Here's how the part is built. I have some questions about the finished solid (model axes, mm). Give positions to 0.01 mm unless a question says otherwise; leave off trailing zeros. Loops run counter-clockwise (first coordinate to the right, second up) from the corner with the lowest first, then second, coordinate; pieces in that order, holes last.
Q1. We'd pull the mould along Y, two halves only. Please class faces 1 (the face through (-1.5, 0.07, 1.97)), 2 (the face through (-5, 0, 4)), 3 (the face through (-1.08, -4.88, 1.53)): +Y half, -Y half, draft (parallel to the pull), parting line (faces both ways), or undercut.
Q2. I need wall thicknesses on line 1 (Y direction, x = 0, z = 3.8); line 2 (Y direction, x = 0, z = 2.75); line 3 (Y direction, x = -0.5, z = 1.2). Which ranges of each line are inside material? Lowest first, please.
Q3. If we section it at B-B (z = 3.25): Please give me the cut outline in (x, y), plus the area to 3 significant figures.
Q4. If we section it at A-A (z = 1.8): Please give me the cut outline in (x, y), plus the area to 3 significant figures.
from build123d import *

# Parameters (mm, degrees)
F0_R     = 2
F0_R_2   = 1.5
F1_DEPTH = 0.25
F0_R_3   = 5
F0_R_4   = 4.5
F2_R     = 5
F2_R_2   = 4.5
F2_R_3   = 2
F2_R_4   = 1.5
F3_DEPTH = 2.75
F4_R     = 5.75
F4_R_2   = 5
F4_R_3   = 1.5
F5_DEPTH = 0.75
F6_R     = 5.75
F6_R_2   = 4.5
F6_R_3   = 2
F6_R_4   = 1.5
F7_DEPTH = 0.25
F8_SIZE  = 0.1


with BuildPart() as f1:
    # F0 (on Top) → F1 (new body)
    with BuildSketch(Plane.XY):
        Circle(F0_R)
        Circle(F0_R_2, mode=Mode.SUBTRACT)
    extrude(amount=F1_DEPTH)



with BuildPart() as f1b:
    # F0 (on Top) → F1, piece 2 (new body)
    with BuildSketch(Plane.XY):
        Circle(F0_R_3)
        Circle(F0_R_4, mode=Mode.SUBTRACT)
    extrude(amount=F1_DEPTH)


with BuildPart() as f1_1:
    add(f1.part)

    add(f1b.part)  # F3 merges F1b
    # F2 (on face) → F3 (join)
    with BuildSketch(Plane.XY.offset(0.25)):
        Circle(F2_R)
        Circle(F2_R_2, mode=Mode.SUBTRACT)
        Circle(F2_R_2)
        Circle(F2_R_3, mode=Mode.SUBTRACT)
        Circle(F2_R_3)
        Circle(F2_R_4, mode=Mode.SUBTRACT)
    extrude(amount=F3_DEPTH)

    # F4 (on face) → F5 (join)
    with BuildSketch(Plane.XY.offset(3)):
        Circle(F4_R)
        Circle(F4_R_2, mode=Mode.SUBTRACT)
        Circle(F4_R_2)
        Circle(F4_R_3, mode=Mode.SUBTRACT)
    extrude(amount=F5_DEPTH)

    # F6 (on face) → F7 (join)
    with BuildSketch(Plane.XY.offset(3.75)):
        Circle(F6_R)
        Circle(F6_R_2, mode=Mode.SUBTRACT)
        Circle(F6_R_3)
        Circle(F6_R_4, mode=Mode.SUBTRACT)
    extrude(amount=F7_DEPTH)

    # F8
    f8_edges = [f1_1.edges().sort_by_distance(p)[0] for p in [
        (-5, 0, 0),
        (-5.75, 0, 3),
        (-5.75, 0, 4),
        (-4.5, 0, 4),
        (-4.5, 0, 0.25),
        (-2, 0, 0),
        (-1.5, 0, 0),
        (-2, 0, 4),
        (-1.5, 0, 4),
    ]]
    chamfer(f8_edges, length=F8_SIZE)


solid = f1_1.part
Check sheet entries:
1. face 1: undercut
1. face 2: draft
1. face 3: parting line
2. line 1: y = -5.75 to -4.5, -2 to -1.5, 1.5 to 2, 4.5 to 5.75
2. line 2: y = -5 to -1.5, 1.5 to 5
2. line 3: y = -4.97 to -1.41, 1.41 to 4.97
3. outline: circle Ø11.5 at (0, 0); hole circle Ø3 at (0, 0)
3. area: 96.8 mm2
4. outline: circle Ø10 at (0, 0); hole circle Ø3 at (0, 0)
4. area: 71.5 mm2
